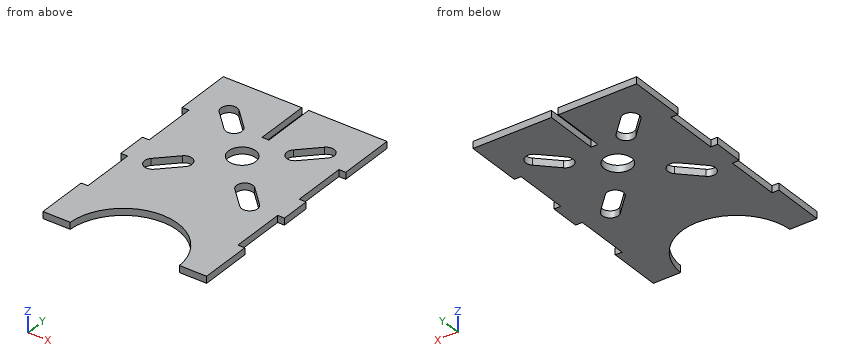
```python
from build123d import *

# Parameters (mm, degrees)
SKETCH9_R           = 6.35
BOSS_EXTRUDE3_DEPTH = 3.175


with BuildPart() as part:
    # Sketch9 → Boss-Extrude3 (new body)
    with BuildSketch(Plane.XY.offset(-50.8)):
        with BuildLine():
            Line((1.5875, 14.934655528), (-1.5875, 14.934655528))
            Line((-1.5875, 14.934655528), (-1.5875, 40.334655528))
            Line((-1.5875, 40.334655528), (-38.1, 40.334655528))
            Line((-38.1, 40.334655528), (-38.1, 13.934655528))
            Line((-38.1, 13.934655528), (-34.925, 13.934655528))
            Line((-34.925, 13.934655528), (-34.925, -11.465344472))
            Line((-34.925, -11.465344472), (-38.1, -11.465344472))
            Line((-38.1, -11.465344472), (-38.1, -25.296741856))
            Line((-38.1, -25.296741856), (-34.925, -25.296741856))
            Line((-34.925, -25.296741856), (-34.925, -50.696741856))
            Line((-34.925, -50.696741856), (-38.1, -50.696741856))
            Line((-38.1, -50.696741856), (-38.1, -75.096741856))
            Line((-38.1, -75.096741856), (-25.429906729, -75.096741856))
            ThreePointArc((-25.429906729, -75.096741856), (0, -50.647180833), (25.429906729, -75.096741856))
            Line((25.429906729, -75.096741856), (38.1, -75.096741856))
            Line((38.1, -75.096741856), (38.1, -50.696741856))
            Line((38.1, -50.696741856), (34.925, -50.696741856))
            Line((34.925, -50.696741856), (34.925, -25.296741856))
            Line((34.925, -25.296741856), (38.1, -25.296741856))
            Line((38.1, -25.296741856), (38.1, -11.465344472))
            Line((38.1, -11.465344472), (34.925, -11.465344472))
            Line((34.925, -11.465344472), (34.925, 13.934655528))
            Line((34.925, 13.934655528), (38.1, 13.934655528))
            Line((38.1, 13.934655528), (38.1, 40.334655528))
            Line((38.1, 40.334655528), (1.5875, 40.334655528))
            Line((1.5875, 40.334655528), (1.5875, 14.934655528))
        make_face()
        with BuildLine():
            ThreePointArc((-21.440764859, -26.794960108), (-26.794960108, -26.794960108), (-26.794960108, -21.440764859))
            Line((-26.794960108, -21.440764859), (-18.385728243, -13.031532993))
            ThreePointArc((-18.385728243, -13.031532993), (-13.031532993, -13.031532993), (-13.031532993, -18.385728243))
            Line((-13.031532993, -18.385728243), (-21.440764859, -26.794960108))
        make_face(mode=Mode.SUBTRACT)
        with BuildLine():
            ThreePointArc((25.020985018, -23.214739949), (25.020985018, -28.568935198), (19.666789768, -28.568935198))
            Line((19.666789768, -28.568935198), (11.257557903, -20.159703333))
            ThreePointArc((11.257557903, -20.159703333), (11.257557903, -14.805508084), (16.611753152, -14.805508084))
            Line((16.611753152, -14.805508084), (25.020985018, -23.214739949))
        make_face(mode=Mode.SUBTRACT)
        with BuildLine():
            ThreePointArc((-25.020985018, 19.666789768), (-25.020985018, 25.020985018), (-19.666789768, 25.020985018))
            Line((-19.666789768, 25.020985018), (-11.257557903, 16.611753152))
            ThreePointArc((-11.257557903, 16.611753152), (-11.257557903, 11.257557903), (-16.611753152, 11.257557903))
            Line((-16.611753152, 11.257557903), (-25.020985018, 19.666789768))
        make_face(mode=Mode.SUBTRACT)
        Circle(SKETCH9_R, mode=Mode.SUBTRACT)
        with BuildLine():
            ThreePointArc((21.440764859, 23.247009927), (26.794960108, 23.247009927), (26.794960108, 17.892814678))
            Line((26.794960108, 17.892814678), (18.385728243, 9.483582813))
            ThreePointArc((18.385728243, 9.483582813), (13.031532993, 9.483582813), (13.031532993, 14.837778062))
            Line((13.031532993, 14.837778062), (21.440764859, 23.247009927))
        make_face(mode=Mode.SUBTRACT)
    extrude(amount=-BOSS_EXTRUDE3_DEPTH)


solid = part.part
```
Verification items for the finished model (mm, model axes). Give positions to 0.01 mm unless a question says otherwise; leave off trailing zeros. Loops run counter-clockwise (first coordinate to the right, second up) from the corner with the lowest first, then second, coordinate; pieces in that order, holes last.
1. Section check C-C, the plane z = -51.8. Count the separate pieces of the cut face and the enclosed holes in it, then the cut area to 3 significant figures.
2. Section check B-B, the plane y = 0. Enter the section's corners in (x, z) (3 decimals).
3. Thickness scan on line 1 (X direction, y = 35.5, z = -53.25); line 2 (Y direction, x = 0, z = -51.9); line 3 (Y direction, x = -14.5, z = -51.9). Record the ranges inside material, lowest first.
4. Go/stop test with a flat-tipped pin: pin 1 Ø1 at (y, z) = (-39, -52) entering from -X (3 decimals). Record where the tip stops, or that it passes through.
5. Section check D-D, the plane x = -8.5. Enter the section's corners in (y, z) (3 decimals), then the cut area to 3 significant figures.
6. Section check A-A, the plane x = 0. Enter the section's corners in (y, z) (3 decimals).
Geometry says:
1. separate pieces: 1
1. enclosed holes: 5
1. area: 6,760 mm2
2. outline: (-34.925, -53.975) - (-6.35, -53.975) - (-6.35, -50.8) - (-34.925, -50.8) - close; (6.35, -53.975) - (34.925, -53.975) - (34.925, -50.8) - (6.35, -50.8) - close
3. line 1: x = -38.1 to -1.59, 1.59 to 38.1
3. line 2: y = -50.65 to -6.35, 6.35 to 14.93
3. line 3: y = -55.18 to -19.85, -12.12 to 10.19, 19.85 to 40.33
4. pin 1: stops at x = -34.925
5. outline: (-52.109, -53.975) - (40.335, -53.975) - (40.335, -50.8) - (-52.109, -50.8) - close
5. area: 294 mm2
6. outline: (-50.647, -53.975) - (-6.35, -53.975) - (-6.35, -50.8) - (-50.647, -50.8) - close; (6.35, -53.975) - (14.935, -53.975) - (14.935, -50.8) - (6.35, -50.8) - close
